CAD build for the part. Positions are in the model's coordinates, mm. A direction names the side the tool comes from. Give positions to 0.01 mm unless a question says otherwise; leave off trailing zeros. Order: outer loops, then holes, each group sorted by start corner. A loop starts at its lowest first (then second) coordinate and runs counter-clockwise, first axis right, second up.
```python
from build123d import *

# Parameters (mm, degrees)
PAD_DEPTH       = 20
POCKET_DEPTH    = 20
SKETCH002_W     = 580
SKETCH002_H     = 300
POCKET001_DEPTH = 20


with BuildPart() as part:
    # Sketch → Pad (new body)
    with BuildSketch(Plane.YZ):
        Polygon((-2000, 200), (-2000, 700), (-750, 1120), (0, 1120), (200, 920), (200, 200), (0, 0), (-1800, 0), align=None)
    extrude(amount=PAD_DEPTH)

    # Sketch001 (on Face10 of Pad) → Pocket (cut)
    with BuildSketch(Plane.YZ.offset(20)):
        Polygon((-950, 250), (-1270, 250), (-1420, 100), (-1420, 0), (-800, 0), (-800, 100), align=None)
    extrude(amount=-POCKET_DEPTH, mode=Mode.SUBTRACT)

    # Sketch002 (on Face5 of Pocket) → Pocket001 (cut)
    with BuildSketch(Plane.YZ.offset(20)):
        with Locations((-420, 790)):
            Rectangle(SKETCH002_W, SKETCH002_H)
    extrude(amount=-POCKET001_DEPTH, mode=Mode.SUBTRACT)


solid = part.part
```
Item 1: Two-plate mould, pull along Y, no slides. Class faces 1 (the face through (20, -885, 568)), 2 (the face through (10, -1344, 176)), 3 (the face through (9.86, -1383.75, 907.06)): released by +Y, released by -Y, zero draft, split by the parting line, or undercut.
Item 2: Slice it at C-C (y = -1700). Give the cut face in (x, z).
Item 3: Slice it at B-B (y = -416). Give the cut face in (x, z), and give its area (3 significant figures).
Item 4: Slice it at D-D (y = -920). Give the cut face in (x, z).
Item 5: Drop flat-ended pins along their axis: pin 1 Ø1 at (x, z) = (8.5, 139) entering from +Y; pin 2 Ø6 at (x, y) = (7, -1053) entering from -Z; pin 3 Ø10 at (x, z) = (14.5, 45.5) entering from -Y. Give the stop position or say it passes through.
Item 6: Slice it at A-A (x = 15.25). Give the cut face in (y, z).
Item 7: Tool access for faces 4 (the face through (10, -874, 174)), 5 (the face through (0, -885, 568)): list every direction of +Z, -Z, +X, -X, +Y, -Y with a clear straight run to the whole face (end or side of a thin tool).
Item 8: Wall check: L1, parallel to Z at x = 6.5, y = -295.5; L2, parallel to Y at x = 6.75, z = 77.5; L3, parallel to Y at x = 10, z = 94.5. Give the ranges that are in metal, low to high.
A:
1. face 1: zero draft
1. face 2: undercut
1. face 3: released by -Y
2. outline: (0, 0) - (20, 0) - (20, 800.8) - (0, 800.8) - close
3. outline: (0, 0) - (20, 0) - (20, 640) - (0, 640) - close; (0, 940) - (20, 940) - (20, 1120) - (0, 1120) - close
3. area: 16,400 mm2
4. outline: (0, 220) - (20, 220) - (20, 1062.88) - (0, 1062.88) - close
5. pin 1: stops at y = 139.5
5. pin 2: stops at z = 250
5. pin 3: stops at y = -1850.5
6. outline: (-2000, 200) - (-1800, 0) - (-1420, 0) - (-1420, 100) - (-1270, 250) - (-950, 250) - (-800, 100) - (-800, 0) - (0, 0) - (200, 200) - (200, 920) - (0, 1120) - (-750, 1120) - (-2000, 700) - close; hole (-710, 640) - (-130, 640) - (-130, 940) - (-710, 940) - close
7. face 4: -Z, +X, -X
7. face 5: +Z, -Z, -X, +Y, -Y
8. L1: z = 0 to 640, 940 to 1120
8. L2: y = -1877.5 to -1420, -800 to 77.5
8. L3: y = -1894.5 to -1420, -800 to 94.5
